```python
from build123d import *
from build123d.topology import SkipClean

# Parameters (mm, degrees)
CROQUIS1_R              = 17.225
CROQUIS1_R_2            = 7.1
SALIENTE_EXTRUIR1_DEPTH = 3
SALIENTE_EXTRUIR2_START = 3
CROQUIS5_R              = 9.1
CROQUIS5_R_2            = 7.1
SALIENTE_EXTRUIR2_DEPTH = 3
REDONDEO1_R             = 3
CROQUIS10_R             = 1.25
CORTAR_EXTRUIR1_DEPTH   = 1.1
CROQUIS12_R             = 9.75
CROQUIS12_R_2           = 7.75
SALIENTE_EXTRUIR3_DEPTH = 13.5
CROQUIS14_R             = 0.75
CORTAR_EXTRUIR3_DEPTH   = 12
MATRIZC1_COUNT          = 4
REDONDEO2_R             = 3


with BuildPart() as part:
    # Croquis1 → Saliente-Extruir1 (new body)
    with BuildSketch(Plane(origin=(0, 0, 0), x_dir=(1, 0, 0), z_dir=(0, 1, 0))):
        with Locations(Location((0, 0, 0), (0, 0, 270))):
            Circle(CROQUIS1_R)
        with Locations(Location((0, 0, 0), (0, 0, 270))):
            Circle(CROQUIS1_R_2, mode=Mode.SUBTRACT)
    extrude(amount=SALIENTE_EXTRUIR1_DEPTH)

    # Croquis5 → Saliente-Extruir2 (add)
    with SkipClean():  # the faces are left unmerged after this step: merging them gives an invalid solid
        with BuildSketch(Plane.XZ.offset(SALIENTE_EXTRUIR2_START)):
            with Locations(Location((0, 0, 0), (0, 0, 90))):
                Circle(CROQUIS5_R)
            with Locations(Location((0, 0, 0), (0, 0, 270))):
                Circle(CROQUIS5_R_2, mode=Mode.SUBTRACT)
        extrude(amount=-SALIENTE_EXTRUIR2_DEPTH)

    # Redondeo1
    redondeo1_edges = [part.edges().sort_by_distance(p)[0] for p in [
        (0, 0, -9.1),
    ]]
    fillet(redondeo1_edges, radius=REDONDEO1_R - 0.0001)  # a hair under: the kernel refuses the full size

    # Croquis10 → Cortar-Extruir1 (cut)
    with BuildSketch(Plane.XZ):
        with Locations(Location((0, 15.276030829, 0), (0, 0, 270))):
            Circle(CROQUIS10_R)
        with Locations(Location((3.798994383, 14.79610623, 0), (0, 0, 270))):
            Circle(CROQUIS10_R)
        with Locations(Location((7.359283978, 13.38648786, 0), (0, 0, 270))):
            Circle(CROQUIS10_R)
        with Locations(Location((10.457162694, 11.135747226, 0), (0, 0, 270))):
            Circle(CROQUIS10_R)
        with Locations(Location((12.89797942, 8.185306639, 0), (0, 0, 270))):
            Circle(CROQUIS10_R)
        with Locations(Location((14.528368663, 4.720553133, 0), (0, 0, 270))):
            Circle(CROQUIS10_R)
        with Locations(Location((15.245887072, 0.959189912, 0), (0, 0, 270))):
            Circle(CROQUIS10_R)
        with Locations(Location((15.005450325, -2.862442738, 0), (0, 0, 270))):
            Circle(CROQUIS10_R)
        with Locations(Location((13.822165949, -6.504217584, 0), (0, 0, 270))):
            Circle(CROQUIS10_R)
        with Locations(Location((11.770384051, -9.737308519, 0), (0, 0, 270))):
            Circle(CROQUIS10_R)
        with Locations(Location((8.979025635, -12.358568548, 0), (0, 0, 270))):
            Circle(CROQUIS10_R)
        with Locations(Location((5.623482016, -14.203294263, 0), (0, 0, 270))):
            Circle(CROQUIS10_R)
        with Locations(Location((1.91459434, -15.155574764, 0), (0, 0, 270))):
            Circle(CROQUIS10_R)
        with Locations(Location((-1.91459434, -15.155574764, 0), (0, 0, 270))):
            Circle(CROQUIS10_R)
        with Locations(Location((-5.623482016, -14.203294263, 0), (0, 0, 270))):
            Circle(CROQUIS10_R)
        with Locations(Location((-8.979025635, -12.358568548, 0), (0, 0, 270))):
            Circle(CROQUIS10_R)
        with Locations(Location((-11.770384051, -9.737308519, 0), (0, 0, 270))):
            Circle(CROQUIS10_R)
        with Locations(Location((-13.822165949, -6.504217584, 0), (0, 0, 270))):
            Circle(CROQUIS10_R)
        with Locations(Location((-15.005450325, -2.862442738, 0), (0, 0, 270))):
            Circle(CROQUIS10_R)
        with Locations(Location((-15.245887072, 0.959189912, 0), (0, 0, 270))):
            Circle(CROQUIS10_R)
        with Locations(Location((-14.528368663, 4.720553133, 0), (0, 0, 270))):
            Circle(CROQUIS10_R)
        with Locations(Location((-12.89797942, 8.185306639, 0), (0, 0, 270))):
            Circle(CROQUIS10_R)
        with Locations(Location((-10.457162694, 11.135747226, 0), (0, 0, 270))):
            Circle(CROQUIS10_R)
        with Locations(Location((-7.359283978, 13.38648786, 0), (0, 0, 270))):
            Circle(CROQUIS10_R)
        with Locations(Location((-3.798994383, 14.79610623, 0), (0, 0, 270))):
            Circle(CROQUIS10_R)
    extrude(amount=-CORTAR_EXTRUIR1_DEPTH, mode=Mode.SUBTRACT)

    # Croquis12 → Saliente-Extruir3 (add)
    with BuildSketch(Plane(origin=(0, 3, 0), x_dir=(1, 0, 0), z_dir=(0, 1, 0))):
        with Locations(Location((0, 0, 0), (0, 0, 270))):
            Circle(CROQUIS12_R)
        with Locations(Location((0, 0, 0), (0, 0, 270))):
            Circle(CROQUIS12_R_2, mode=Mode.SUBTRACT)
    extrude(amount=SALIENTE_EXTRUIR3_DEPTH)

    # Croquis14 → Cortar-Extruir3 (cut)
    with BuildSketch(Plane(origin=(0, 0, 0), x_dir=(0, 0, -1), z_dir=(1, 0, 0))):
        with Locations((0, 14.5)):
            Circle(CROQUIS14_R)
    cortar_extruir3 = extrude(amount=-CORTAR_EXTRUIR3_DEPTH, mode=Mode.SUBTRACT)

    # MatrizC1: Cortar-Extruir3 ×4 about axis
    matrizc1_axis = Axis((0, 16.5, 0), (0, -1, 0))
    for i in range(1, MATRIZC1_COUNT):
        add(cortar_extruir3.rotate(matrizc1_axis, i * 360 / MATRIZC1_COUNT), mode=Mode.SUBTRACT)

    # Redondeo2
    redondeo2_edges = [part.edges().sort_by_distance(p)[0] for p in [
        (0, 3, -9.75),
    ]]
    fillet(redondeo2_edges, radius=REDONDEO2_R)


solid = part.part
```
CAD build for the part. Positions are in the model's coordinates, mm. A direction names the side the tool comes from. Coordinates: 2 decimals unless noted, no trailing zeros. Loops run counter-clockwise (first coordinate to the right, second up) from the corner with the lowest first, then second, coordinate; pieces in that order, holes last. Notation, with made-up numbers: (9.5, -33) - (41.5, -33) arc R29 ccw to (41.5, -10) - close; hole circle Ø6 at (85, 28.5). An arc over 180 degrees is marked (long way). Return JSON: item names as keys, results as strings.
1. Drop flat-ended pins along their axis: pin 1 (6 mm diameter, centred on y = 12, z = 11.5, fed in from -X); pin 2 (4 mm diameter, centred on x = 1, y = 6.5, fed in from +Z); pin 3 (6 mm diameter, centred on x = -12, z = -6, fed in from +Y); pin 4 (12 mm diameter, centred on x = -9.5, z = 7.5, fed in from -Y). Give the stop position or say it passes through.
Result:
{"pin 1": "stops at x = -4.78", "pin 2": "stops at z = 10.12", "pin 3": "stops at y = 4.11", "pin 4": "stops at y = -3"}
2. Band-saw the part on B-B (x = 0). State how many separate pieces and enclosed holes the cut face has, and give its area (3 significant figures).
Result:
{"separate pieces": "4", "enclosed holes": "0", "area": "126 mm2"}
3. 3-axis set-ups, long thin cutter, end or side, ignore diameter. For faces 4 (the cylindrical face through (2.3, 9.7, 7.4)), 5 (the flat face through (0, 1.1, 15)): which of +Z, -Z, +X, -X, +Y, -Y reach the whole face in a straight line?
Result:
{"face 4": "+Y", "face 5": "-Y"}
4. Mould opens along X. For faces 1 (the flat face through (13, 1.1, 8)), 2 (the cylindrical face through (8.718, 15.244, -0.098)), 3 (the cylindrical face through (-11.677, 0.542, 11.407)) say: released by +X, released by -X, zero draft, split by the parting line, or undercut.
Result:
{"face 1": "undercut", "face 2": "zero draft", "face 3": "undercut"}
5. Band-saw the part on C-C (z = 15.5). Give the cut face in (x, y).
Result:
{"outline": "(-7.51, 0) - (-4.83, 0) - (-4.83, 1.1) - (-2.77, 1.1) - (-2.77, 0) - (-1.23, 0) - (-1.23, 1.1) - (1.23, 1.1) - (1.23, 0) - (2.77, 0) - (2.77, 1.1) - (4.83, 1.1) - (4.83, 0) - (7.51, 0) - (7.51, 3) - (-7.51, 3) - close"}
6. Band-saw the part on D-D (y = 8). Give the cut face in (x, z).
Result:
{"outline": "circle Ø19.5 at (0, 0); hole circle Ø15.5 at (0, 0)"}
7. Probe L1, parallel to Y at x = -4, z = -12; L2, parallel to X at y = 14.5, z = 8.85; L3, parallel to Y at x = 8, z = -12. List the from-to ranges inside material, lowest first. Write a range as from..to.
Result:
{"L1": "y = 0..3", "L2": "x = -4.09..-0.75, 0.75..4.09", "L3": "y = 1.1..3"}
8. Band-saw the part on A-A (y = 14.5). Give the cut face in (x, z).
Result:
{"outline": "(-9.72, -0.75) arc R9.75 ccw to (-0.75, -9.72) - (-0.75, -7.71) arc R7.75 cw to (-7.71, -0.75) - close; (-9.72, 0.75) - (-7.71, 0.75) arc R7.75 cw to (-0.75, 7.71) - (-0.75, 9.72) arc R9.75 ccw to start; (0.75, -9.72) arc R9.75 ccw to (9.72, -0.75) - (7.71, -0.75) arc R7.75 cw to (0.75, -7.71) - close; (0.75, 7.71) arc R7.75 cw to (7.71, 0.75) - (9.72, 0.75) arc R9.75 ccw to (0.75, 9.72) - close"}
